Could you check a few things on this model? Use its own coordinates, in mm. Face numbers are marked on the shaded views. A direction names the side the tool comes from. Coordinates: 2 decimals unless noted, no trailing zeros. Write each loop counter-clockwise with the first axis right and the second up, starting at its lowest first coordinate (ties: lowest second). Pieces come first, ordered by that corner, then holes.
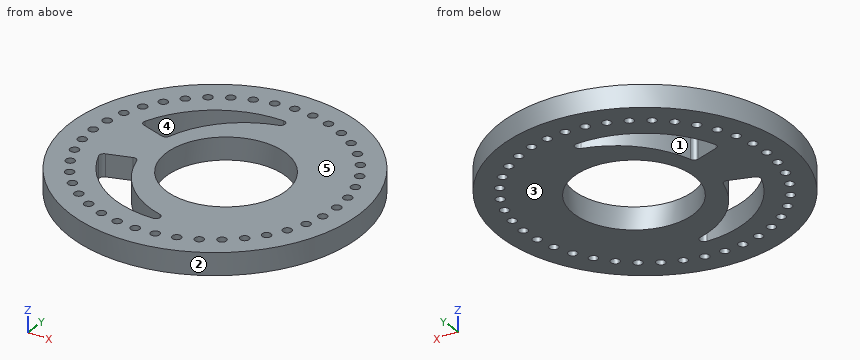
```python
from build123d import *

# Parameters (mm, degrees)
SKETCH_5_R      = 65
SKETCH_5_R_2    = 2
SKETCH_5_R_3    = 27
EXTRUDE_3_DEPTH = 10
FILLET_1_R      = 2


with BuildPart() as part:
    # 草图5 → 凸台-拉伸3 (new body)
    with BuildSketch(Plane.XY):
        Circle(SKETCH_5_R)
        with Locations((55, 0)):
            Circle(SKETCH_5_R_2, mode=Mode.SUBTRACT)
        with Locations((54.322858733, -8.603895577)):
            Circle(SKETCH_5_R_2, mode=Mode.SUBTRACT)
        with Locations((52.308108396, -16.995934691)):
            Circle(SKETCH_5_R_2, mode=Mode.SUBTRACT)
        with Locations((49.00535883, -24.969477486)):
            Circle(SKETCH_5_R_2, mode=Mode.SUBTRACT)
        with Locations((44.495934691, -32.328188876)):
            Circle(SKETCH_5_R_2, mode=Mode.SUBTRACT)
        with Locations((38.890872965, -38.890872965)):
            Circle(SKETCH_5_R_2, mode=Mode.SUBTRACT)
        with Locations((32.328188876, -44.495934691)):
            Circle(SKETCH_5_R_2, mode=Mode.SUBTRACT)
        with Locations((24.969477486, -49.00535883)):
            Circle(SKETCH_5_R_2, mode=Mode.SUBTRACT)
        with Locations((16.995934691, -52.308108396)):
            Circle(SKETCH_5_R_2, mode=Mode.SUBTRACT)
        with Locations((8.603895577, -54.322858733)):
            Circle(SKETCH_5_R_2, mode=Mode.SUBTRACT)
        with Locations((0, -55)):
            Circle(SKETCH_5_R_2, mode=Mode.SUBTRACT)
        with Locations((-8.603895577, -54.322858733)):
            Circle(SKETCH_5_R_2, mode=Mode.SUBTRACT)
        with Locations((-16.995934691, -52.308108396)):
            Circle(SKETCH_5_R_2, mode=Mode.SUBTRACT)
        with Locations((-24.969477486, -49.00535883)):
            Circle(SKETCH_5_R_2, mode=Mode.SUBTRACT)
        with Locations((-32.328188876, -44.495934691)):
            Circle(SKETCH_5_R_2, mode=Mode.SUBTRACT)
        with Locations((-38.890872965, -38.890872965)):
            Circle(SKETCH_5_R_2, mode=Mode.SUBTRACT)
        with Locations((-44.495934691, -32.328188876)):
            Circle(SKETCH_5_R_2, mode=Mode.SUBTRACT)
        with Locations((-49.00535883, -24.969477486)):
            Circle(SKETCH_5_R_2, mode=Mode.SUBTRACT)
        with Locations((-52.308108396, -16.995934691)):
            Circle(SKETCH_5_R_2, mode=Mode.SUBTRACT)
        with Locations((-54.322858733, -8.603895577)):
            Circle(SKETCH_5_R_2, mode=Mode.SUBTRACT)
        with Locations((-55, 0)):
            Circle(SKETCH_5_R_2, mode=Mode.SUBTRACT)
        with Locations((-54.322858733, 8.603895577)):
            Circle(SKETCH_5_R_2, mode=Mode.SUBTRACT)
        with Locations((-52.308108396, 16.995934691)):
            Circle(SKETCH_5_R_2, mode=Mode.SUBTRACT)
        with Locations((-49.00535883, 24.969477486)):
            Circle(SKETCH_5_R_2, mode=Mode.SUBTRACT)
        with Locations((-44.495934691, 32.328188876)):
            Circle(SKETCH_5_R_2, mode=Mode.SUBTRACT)
        with Locations((-38.890872965, 38.890872965)):
            Circle(SKETCH_5_R_2, mode=Mode.SUBTRACT)
        with Locations((-32.328188876, 44.495934691)):
            Circle(SKETCH_5_R_2, mode=Mode.SUBTRACT)
        with Locations((-24.969477486, 49.00535883)):
            Circle(SKETCH_5_R_2, mode=Mode.SUBTRACT)
        with Locations((-16.995934691, 52.308108396)):
            Circle(SKETCH_5_R_2, mode=Mode.SUBTRACT)
        with Locations((-8.603895577, 54.322858733)):
            Circle(SKETCH_5_R_2, mode=Mode.SUBTRACT)
        with Locations((0, 55)):
            Circle(SKETCH_5_R_2, mode=Mode.SUBTRACT)
        with Locations((8.603895577, 54.322858733)):
            Circle(SKETCH_5_R_2, mode=Mode.SUBTRACT)
        with Locations((16.995934691, 52.308108396)):
            Circle(SKETCH_5_R_2, mode=Mode.SUBTRACT)
        with Locations((24.969477486, 49.00535883)):
            Circle(SKETCH_5_R_2, mode=Mode.SUBTRACT)
        with Locations((32.328188876, 44.495934691)):
            Circle(SKETCH_5_R_2, mode=Mode.SUBTRACT)
        with Locations((38.890872965, 38.890872965)):
            Circle(SKETCH_5_R_2, mode=Mode.SUBTRACT)
        with Locations((44.495934691, 32.328188876)):
            Circle(SKETCH_5_R_2, mode=Mode.SUBTRACT)
        with Locations((49.00535883, 24.969477486)):
            Circle(SKETCH_5_R_2, mode=Mode.SUBTRACT)
        with Locations((52.308108396, 16.995934691)):
            Circle(SKETCH_5_R_2, mode=Mode.SUBTRACT)
        with Locations((54.322858733, 8.603895577)):
            Circle(SKETCH_5_R_2, mode=Mode.SUBTRACT)
        with Locations((5, 0)):
            Circle(SKETCH_5_R_3, mode=Mode.SUBTRACT)
        with BuildLine():
            Line((-42.797543233, 13.905764747), (-28.480319158, 9.253816649))
            ThreePointArc((-28.480319158, 9.253816649), (-12.826252178, 33.752847264), (14.913461538, 42.456903619))
            ThreePointArc((14.913461538, 42.456903619), (-19.954257333, 40.333951136), (-42.797543233, 13.905764747))
        make_face(mode=Mode.SUBTRACT)
        with BuildLine():
            Line((-42.797543233, -13.905764747), (-28.480319158, -9.253816649))
            ThreePointArc((-28.480319158, -9.253816649), (-12.826252178, -33.752847264), (14.913461538, -42.456903619))
            ThreePointArc((14.913461538, -42.456903619), (-19.954257333, -40.333951136), (-42.797543233, -13.905764747))
        make_face(mode=Mode.SUBTRACT)
    extrude(amount=EXTRUDE_3_DEPTH)

    # 圆角1
    fillet_1_edges = [part.edges().sort_by_distance(p)[0] for p in [
        (-42.797543233, 13.905764747, 5),
        (-28.480319158, 9.253816649, 5),
        (14.913461538, 42.456903619, 5),
        (-28.480319158, -9.253816649, 5),
        (-42.797543233, -13.905764747, 5),
        (14.913461538, -42.456903619, 5),
    ]]
    fillet(fillet_1_edges, radius=FILLET_1_R)


solid = part.part
```
Item 1: I want a section at B-B, the plane x = -5. List the corners of the cut face in (y, z) for me, then the cut area to 3 significant figures.
Item 2: Which directions (+Z, -Z, +X, -X, +Y, -Y) give clear straight access to the entire face, cutting with the end or side of a thin tool? Please do the marked faces 4 and 5.
Item 3: If I drill on line 1 along X through (y, z) = (-34, 6.75); line 2 along Y through (x, z) = (0, 5.75); line 3 along Y through (x, z) = (-53.5, 6.25), over which ranges is the centre line in solid material (lowest first)?
Item 4: Will these pins go through, and if not, where does the flat tip stop? pin 1 Ø3.5 at (x, y) = (44.5, 32.33) entering from -Z; pin 2 Ø5 at (x, z) = (45, 6) entering from -Y; pin 3 Ø3 at (x, z) = (-15.5, 3) entering from +Y; pin 4 Ø6 at (x, z) = (-8.5, 1) entering from +Y.
Item 5: I want a section at C-C, the plane z = 5. Count the separate pieces of the cut face and the enclosed holes in it, then the cut area to 3 significant figures.
Item 6: If we mould it in two halves opening along Y, with no side actions, what happens to the marked faces 1, 2 and 3? For each: released by +Y, released by -Y, zero draft, split by the parting line, or undercut.
Item 7: I want a section at A-A, the plane y = 0. List the corners of the cut face in (x, z) for me, then the cut area to 3 significant figures.
Taken from the geometry:
1. outline: (-64.81, 0) - (-44.72, 0) - (-44.72, 10) - (-64.81, 10) - close; (-38.5, 0) - (-25.08, 0) - (-25.08, 10) - (-38.5, 10) - close; (25.08, 0) - (38.5, 0) - (38.5, 10) - (25.08, 10) - close; (44.72, 0) - (64.81, 0) - (64.81, 10) - (44.72, 10) - close
1. area: 670 mm2
2. face 4: +Z, -Z
2. face 5: +Z, +X, -X, +Y, -Y
3. line 1: x = -55.4 to -45.59, -43.4 to -29.48, -12.5 to 43.4, 45.59 to 55.4
3. line 2: y = -65 to -57, -53 to -45, -40.46 to -26.53, 26.53 to 40.46, 45 to 53, 57 to 65
3. line 3: y = -36.92 to -18.6, -15.39 to -10.43, -6.78 to -1.32, 1.32 to 6.78, 10.43 to 15.39, 18.6 to 36.92
4. pin 1: passes through
4. pin 2: stops at y = -49.18
4. pin 3: stops at y = 63.47
4. pin 4: stops at y = 64.77
5. separate pieces: 1
5. enclosed holes: 43
5. area: 9,390 mm2
6. face 1: undercut
6. face 2: split by the parting line
6. face 3: zero draft
7. outline: (-65, 0) - (-57, 0) - (-57, 10) - (-65, 10) - close; (-53, 0) - (-22, 0) - (-22, 10) - (-53, 10) - close; (32, 0) - (53, 0) - (53, 10) - (32, 10) - close; (57, 0) - (65, 0) - (65, 10) - (57, 10) - close
7. area: 680 mm2
